Build history of the part. All positions in model axes, mm. Round coordinates to 2 decimals unless told otherwise and drop trailing zeros. Write each loop counter-clockwise with the first axis right and the second up, starting at its lowest first coordinate (ties: lowest second). Pieces come first, ordered by that corner, then holes.
from build123d import *

# Parameters (mm, degrees)
F1_DEPTH = 125.1
F2_W     = 44
F2_H     = 8.367
F3_DEPTH = 125.1
F4_R     = 8
F5_DEPTH = 4


with BuildPart() as f1:
    # F0 (on Front) → F1 (new body)
    with BuildSketch(Plane.XZ):
        with BuildLine():
            ThreePointArc((-37.5, 0), (0, 37.5), (37.5, 0))
            Line((37.5, 0), (45.5, 0))
            ThreePointArc((45.5, 0), (0, 45.5), (-45.5, 0))
            Line((-45.5, 0), (-37.5, 0))
        make_face()
    extrude(amount=F1_DEPTH)

    # F2 (on Front) → F3 (cut)
    with BuildSketch(Plane.XZ):
        with Locations((0, 44.6835)):
            Rectangle(F2_W, F2_H)
    extrude(amount=F3_DEPTH, mode=Mode.SUBTRACT)

    # F4 (on face) → F5 (cut)
    with BuildSketch(Plane.XY.offset(40.5)):
        with Locations((0, -62.5)):
            Circle(F4_R)
    extrude(amount=-F5_DEPTH, mode=Mode.SUBTRACT)


solid = f1.part
1) Mould opens along Y. For faces 1 (the flat face through (0, -125.1, 40)), 2 (the cylindrical face through (-38.635, -61.674, 24.033)), 3 (the cylindrical face through (4.301, -55.754, 38.595)) say: released by +Y, released by -Y, zero draft, split by the parting line, or undercut.
Results:
face 1: released by -Y
face 2: zero draft
face 3: undercut
2) Pin check, flat tips, straight feed: pin 1 Ø5 at (y, z) = (-18.5, 36.5) entering from +X; pin 2 Ø18.5 at (x, y) = (0, -62.5) entering from -Z; pin 3 Ø1.5 at (x, y) = (-24, -69) entering from -Z. Stop position of each tip, or through.
Results:
pin 1: stops at x = 30.24
pin 2: stops at z = 36.34
pin 3: stops at z = 28.17
3) Slice it at B-B (x = 0). Write the cut outline in (y, z), plus the area to 3 significant figures.
Results:
outline: (-125.1, 37.5) - (-70.5, 37.5) - (-70.5, 40.5) - (-125.1, 40.5) - close; (-54.5, 37.5) - (0, 37.5) - (0, 40.5) - (-54.5, 40.5) - close
area: 327 mm2
4) Slice it at D-D (y = -89). Write the cut outline in (x, z), plus the area to 3 significant figures.
Results:
outline: (-45.5, 0) - (-37.5, 0) arc R37.5 cw to (37.5, 0) - (45.5, 0) arc R45.5 ccw to (20.74, 40.5) - (-20.74, 40.5) arc R45.5 ccw to start
area: 903 mm2
5) Wall check: L1, parallel to Y at x = 0, z = 39; L2, parallel to X at y = -62.5, z = 39; L3, parallel to X at y = -62, z = 37. Give the ranges that are in metal, low to high.
Results:
L1: y = -125.1 to -70.5, -54.5 to 0
L2: x = -23.44 to -8, 8 to 23.44
L3: x = -26.48 to -7.98, 7.98 to 26.48
6) Slice it at C-C (z = 29.5). Write the cut outline in (x, y), plus the area to 3 significant figures.
Results:
outline: (-34.64, -125.1) - (-23.15, -125.1) - (-23.15, 0) - (-34.64, 0) - close; (23.15, -125.1) - (34.64, -125.1) - (34.64, 0) - (23.15, 0) - close
area: 2,870 mm2
7) Slice it at A-A (y = -62.5). Write the cut outline in (x, z).
Results:
outline: (-45.5, 0) - (-37.5, 0) arc R37.5 cw to (-8, 36.64) - (-8, 40.5) - (-20.74, 40.5) arc R45.5 ccw to start; (8, 36.64) arc R37.5 cw to (37.5, 0) - (45.5, 0) arc R45.5 ccw to (20.74, 40.5) - (8, 40.5) - close
